```python
from build123d import *

# Parameters (mm, degrees)
F1_DEPTH  = 15
F2_R      = 1
F3_R      = 1
F4_R      = 1
F6_DEPTH  = 25
F8_DEPTH  = 25
F9_W      = 2
F9_H      = 19
F10_DEPTH = 5


with BuildPart() as f1:
    # F0 (on Right) → F1 (new body)
    with BuildSketch(Plane.YZ):
        Polygon((-24.8861957348, -43.0121933088), (-39.0283313585, -28.8700576851), (-40.4425449209, -30.2842712475), (-24.8861957348, -45.8406204336), (31.0965603225, 10.1421356237), (31.0965603225, -45.8406204336), (33.0965603225, -45.8406204336), (33.0965603225, 12.1421356237), (31.6823467601, 13.5563491861), align=None)
    extrude(amount=F1_DEPTH)

    # F2
    f2_edges = [f1.edges().sort_by_distance(p)[0] for p in [
        (7.5, -24.886196, -43.012193),
    ]]
    fillet(f2_edges, radius=F2_R)

    # F3
    f3_edges = [f1.edges().sort_by_distance(p)[0] for p in [
        (7.5, 31.09656, 10.142136),
    ]]
    fillet(f3_edges, radius=F3_R)

    # F4
    f4_edges = [f1.edges().sort_by_distance(p)[0] for p in [
        (7.5, -24.886196, -45.84062),
        (7.5, 31.682347, 13.556349),
        (7.5, 33.09656, 12.142136),
    ]]
    fillet(f4_edges, radius=F4_R)

    # F5 (on face) → F6 (join)
    with BuildSketch(Plane.YZ.offset(15)):
        Polygon((-25.593302516, -42.3050865276), (-39.0283313585, -28.8700576851), (-40.4425449209, -30.2842712475), (-27.0075160784, -43.71930009), align=None)
    extrude(amount=F6_DEPTH)

    # F7 (on face) → F8 (join)
    with BuildSketch(Plane(origin=(0, 0, 0), x_dir=(0, -1, 0), z_dir=(-1, 0, 0))):
        Polygon((40.4425449209, -30.2842712475), (39.0283313585, -28.8700576851), (25.593302516, -42.3050865276), (27.0075160784, -43.71930009), align=None)
    extrude(amount=F8_DEPTH)

    # F9 (on face) → F10 (join)
    with BuildSketch(Plane(origin=(0, -33.9491945218, -33.9491945218), x_dir=(-1, 0, 0), z_dir=(0, 0.7071067812, 0.7071067812))):
        with Locations((24, -2.3170158004)):
            Rectangle(F9_W, F9_H)
        with Locations((-39, -2.3170158004)):
            Rectangle(F9_W, F9_H)
    extrude(amount=F10_DEPTH)


solid = f1.part
```
Model file for the job. Use its own axes, mm. A direction names the side the tool comes from. Give positions to 0.01 mm unless a question says otherwise; leave off trailing zeros. Write each loop counter-clockwise with the first axis right and the second up, starting at its lowest first coordinate (ties: lowest second). Pieces come first, ordered by that corner, then holes. Notation, with made-up numbers: (-26.75, 71.5) - (27.25, 71.5) arc R16 ccw to (27.25, 86.5) - close; hole circle Ø10 at (58, -32.75). An arc over 180 degrees is marked (long way). One line per question, with ' | ' between items. Start each with the question number.
(1) 3-axis set-ups, long thin cutter, end or side, ignore diameter. For faces 4 (the face through (7.395, 3.784, -14.342)), 5 (the face through (7.9, -32.4, -35.5)), 6 (the face through (38, -30, -34)), 7 (the face through (7.395, 2.23, -18.724)): which of +Z, -Z, +X, -X, +Y, -Y reach the whole face in a straight line?
(2) Slice it at D-D on y = 18. Write the cut outline in (x, z).
(3) Wall check: line 1 along Y through (x, z) = (5, -38); line 2 along Y through (x, z) = (0.5, 4); line 3 along Y through (x, z) = (9, -25.5). Give the ranges that are in metal, low to high. Write a range as from..to.
(4) Two-plate mould, pull along Y, no slides. Class faces 1 (the face through (7, 33.097, -17)), 2 (the face through (15, 7, -12)), 3 (the face through (7, 31.097, -19)): +Y half, -Y half, draft (parallel to the pull), parting line (faces both ways), or undercut.
(5) Slice it at A-A on z = -11. Write the cut outline in (x, y).
(6) Pin check, flat tips, straight feed: P1, Ø2, axis at x = -10, z = -37.5, coming from the -Y side; P2, Ø6, axis at y = -18, z = -34, coming from the -X side; P3, Ø5, axis at x = 24, z = -38, coming from the +Y side. Stop position of each tip, or through.
(7) Slice it at C-C on z = -32.5. Write the cut outline in (x, y).
(8) Slice it at B-B on x = 1. Write the cut outline in (y, z).
Results below:
1) face 4: +Z, +X, -X | face 5: +Z | face 6: +Z, +Y | face 7: -Z, +X, -X
2) outline: (0, -2.95) - (15, -2.95) - (15, -0.13) - (0, -0.13) - close
3) line 1: -32.73..-29.9, -19.87..-17.05, 31.1..33.1 | line 2: 22.13..24.95, 31.1..33.1 | line 3: -7.37..-4.55, 31.1..33.1
4) face 1: +Y half | face 2: draft | face 3: undercut
5) outline: (0, 7.13) - (15, 7.13) - (15, 9.95) - (0, 9.95) - close; (0, 31.1) - (15, 31.1) - (15, 33.1) - (0, 33.1) - close
6) P1: y = -34.23 | P2: x = 0 | P3: y = -27.4
7) outline: (-25, -38.23) - (40, -38.23) - (40, -28.33) - (38, -28.33) - (38, -35.4) - (-23, -35.4) - (-23, -28.33) - (-25, -28.33) - close; (0, -14.37) - (15, -14.37) - (15, -11.55) - (0, -11.55) - close; (0, 31.1) - (15, 31.1) - (15, 33.1) - (0, 33.1) - close
8) outline: (-40.44, -30.28) - (-25.59, -45.13) arc R1 ccw to (-24.18, -45.13) - (29.39, 8.44) arc R1 cw to (31.1, 7.73) - (31.1, -45.84) - (33.1, -45.84) - (33.1, 11.73) arc R1 ccw to (32.8, 12.44) - (32.39, 12.85) arc R1 ccw to (30.98, 12.85) - (-24.18, -42.31) arc R1 cw to (-25.59, -42.31) - (-39.03, -28.87) - close
